Autodesk Inventor part; units mm, degrees
ref_plane "YZ Plane" through (0, 0, 0) normal (1, 0, 0) x (0, 1, 0)
ref_plane "XZ Plane" through (0, 0, 0) normal (0, 1, 0) x (-1, 0, 0)
ref_plane "XY Plane" through (0, 0, 0) normal (0, 0, 1) x (1, 0, 0)
sketch "Náčrt1" plane through (0, 0, 0) normal (0, 0, 1) x (1, 0, 0)
  line L0 (0, 0) -> (14.198, 0)
  line L1 (0, 19.135) -> (0, 30)
  line L2 (0, 30) -> (14, 30)
  line L3 (14, 30) -> (14, 23.8859)
  line L4 (3.5, 18.76) -> (2.3, 18.76)
  arc A0 (3.5, 18.76) -> (13.7308, 23.2033) centre (3.5, 32.76) ccw
  arc A1 (13.7308, 23.2033) -> (14, 23.8859) centre (13, 23.8859) ccw
  line L5 (0.3, 18.835) -> (1.0738, 18.835)
  line L6 (1.0738, 18.835) -> (2.3, 18.76)
  arc A2 (0, 19.135) -> (0.3, 18.835) centre (0.3, 19.135) ccw
  point P0 (0, 18.835)
  dimension "d0" = 60
  dimension "d1" = 37.52
  dimension "d4" = 14
  dimension "d18" = 1
  dimension "d21" = 14
  dimension "d25" = 10.5
  dimension "d26" = 1.2
  dimension "d27" = 37.67
  dimension "d28" = 3.5
  dimension "d29" = 0.3
  dimension "d32" = 5.1259
revolve "Rotace1" add sketch "Náčrt1" angle 360 about axis through (0, 0, 0) along (1, 0, 0)
chamfer "Zkosení1" distance 1 angle 45 1 edges at (0, -30, 0)
chamfer "Zkosení2" distance 0.5 angle 45 1 edges at (14, -30, 0)
equation "\"Rozmer_B\" = 0"
equation "\"Rozmer_C\" = 0"
equation "\"Rozmer_D\" = d21"
properties part number "NA-45-h-Crown-129" material "19 436.4"
Check sheet for the modelled part. Datum: model origin and axes. Units: mm. Give positions to 0.01 mm unless a question says otherwise; leave off trailing zeros. Order: outer loops, then holes, each group sorted by start corner. A loop starts at its lowest first (then second) coordinate and runs counter-clockwise, first axis right, second up. Notation, with made-up numbers: (72, -21.5) -> (97, -21.5) arc R16 ccw to (97, 2.5) -> close; hole circle Ø3 at (7.5, 51.5). An arc over 180 degrees is marked (long way). Use CSV: the item, a comma, the result in double quotes. Start each with the question number.
1) Mould release check, pull along Z, two halves, no side actions. Record for faces 1 (the face through (0.69, 17.4, -7.21)), 2 (the face through (7.34, -29.97, 1.32)), 3 (the face through (14, -2, -24)): released by +Z, released by -Z, zero draft, split by the parting line, or undercut.
2) Material ranges on line 1 (Z direction, x = 0.5, y = 0) (3 decimals); line 2 (Z direction, x = 3, y = 0); line 3 (Y direction, x = 11.75, z = 15), recorded low to high. Write a range as from..to.
3) Sectioned sample at A-A, the plane z = 0. Record the boundary of the cut face in (x, y) (3 decimals), plus the area to 3 significant figures.
4) Go/stop test with flat-tipped pins: P1, Ø1, axis at x = 9, z = -3, coming from the +Y side; P2, Ø8, axis at x = 3, y = -10.5, coming from the +Z side; P3, Ø1.5, axis at x = 9.5, y = 10.5, coming from the -Z side; P4, Ø5, axis at y = 1, z = -17.5, coming from the -X side. Record where each tip stops, or that it passes through.
5) Sectioned sample at C-C, the plane x = 10.25. Record the boundary of the cut face in (y, z).
6) Sectioned sample at D-D, the plane x = 6. Record the boundary of the cut face in (y, z).
Recorded:
1,face 1,"undercut"
1,face 2,"split by the parting line"
1,face 3,"zero draft"
2,line 1,"-29.5..-18.835, 18.835..29.5"
2,line 2,"-30..-18.76, 18.76..30"
2,line 3,"-25.98..-15.33, 15.33..25.98"
3,outline,"(0, -29) -> (1, -30) -> (13.5, -30) -> (14, -29.5) -> (14, -23.886) arc R1 ccw to (13.731, -23.203) arc R14 ccw to (3.5, -18.76) -> (2.3, -18.76) -> (1.074, -18.835) -> (0.3, -18.835) arc R0.3 ccw to (0, -19.135) -> close; (0, 19.135) arc R0.3 ccw to (0.3, 18.835) -> (1.074, 18.835) -> (2.3, 18.76) -> (3.5, 18.76) arc R14 ccw to (13.731, 23.203) arc R1 ccw to (14, 23.886) -> (14, 29.5) -> (13.5, 30) -> (1, 30) -> (0, 29) -> close"
3,area,"283 mm2"
4,P1,"y = 29.9"
4,P2,"z = 29.29"
4,P3,"z = -28.37"
4,P4,"x = 0"
5,outline,"circle Ø60 at (0, 0); hole circle Ø40.99 at (0, 0)"
6,outline,"circle Ø60 at (0, 0); hole circle Ø37.97 at (0, 0)"
